Build history of the part. All positions in model axes, mm. A direction names the side the tool comes from. Coordinates: 2 decimals unless noted, no trailing zeros. Loops run counter-clockwise (first coordinate to the right, second up) from the corner with the lowest first, then second, coordinate; pieces in that order, holes last. Notation, with made-up numbers: (19.5, -33) -> (45.5, -33) arc R15 cw to (45.5, -29) -> close; hole circle Ø10 at (2, 41). An arc over 180 degrees is marked (long way). One line per item, written item: value. Start each with the question number.
Autodesk Inventor part; units mm, degrees
ref_plane "YZ Plane" through (0, 0, 0) normal (1, 0, 0) x (0, 1, 0)
ref_plane "XZ Plane" through (0, 0, 0) normal (0, 1, 0) x (-1, 0, 0)
ref_plane "XY Plane" through (0, 0, 0) normal (0, 0, 1) x (1, 0, 0)
sketch "Boceto1" plane through (0, 0, 0) normal (0, 1, 0) x (-1, 0, 0)
  line L0 (0, 0) -> (0, -22)
  line L1 (0, -22) -> (0, -23)
  line L2 (0, 0) -> (15, 0)
  line L3 (0, -23) -> (15, -23)
  line L4 (15, -23) -> (15, -27)
  line L5 (15, -27) -> (-4, -27)
  line L6 (-4, -27) -> (-4, 0)
  line L7 (-4, 0) -> (-4, 4)
  line L8 (-4, 4) -> (15, 4)
  line L9 (15, 4) -> (15, 0)
  line L10 (15, 4) -> (10, 4)
  line L11 (10, 4) -> (-4, 2)
  line L12 (15, -27) -> (10, -27)
  line L13 (10, -27) -> (-4, -25.6809)
  dimension "d0" = 22
  dimension "d1" = 1
  dimension "d2" = 15
  dimension "d3" = 15
  dimension "d4" = 4
  dimension "d5" = 19
  dimension "d6" = 4
  dimension "d7" = 5
  dimension "d8" = 5
extrude "Extrusión1" add sketch "Boceto1" along normal blind 12 contours L0 L1 L3 L4 L5 L13 L6 L7 L11 L8 L9 L2
sketch "Boceto2" plane through (-15, 0, 0) normal (-1, 0, 0) x (0, 0, 1)
  line L0 (4, 0) -> (4, 12)
  line L1 (4, 6) -> (-27, 6)
  line L2 (-27, 0) -> (-27, 12)
  line L3 (4, 6) -> (3, 6)
  circle A0 centre (3, 6) radius 1
  line L4 (-27, 6) -> (-26, 6)
  circle A1 centre (-26, 6) radius 1
  point P0 (0, 0)
  dimension "d11" = 1
  dimension "d12" = 1
extrude "Extrusión2" cut sketch "Boceto2" against normal blind 12
sketch "Boceto3" plane through (0, 12, 0) normal (0, 1, 0) x (1, 0, 0)
  line L0 (-10, -4) -> (4, -2)
  line L1 (0, -2.5714) -> (-15, -2.5714)
  line L2 (-15, -2) -> (-3, -2)
  line L3 (-15, -2.5714) -> (-13, -2.5714)
  line L4 (-13, -2.5714) -> (-13, -4)
  line L5 (-15, -4) -> (-10, -4)
  line L6 (-13, -4) -> (-10.0485, -4)
  line L7 (-10.0485, -4) -> (0, -2.5714)
  line L8 (-10, 27) -> (-15, 27)
  line L9 (-15, 27) -> (-13, 27)
  line L10 (-13, 27) -> (-13, 25.6179)
  line L11 (-13, 25.6179) -> (-3.0681, 25.6179)
  line L12 (-10, 27) -> (-3, 26.3405)
  line L13 (-3.0681, 25.6179) -> (-3, 26.3405)
  line L14 (-3, 26.3405) -> (-13, 27)
  line L15 (-13, 27) -> (-10, 27)
  line L16 (-10, 27) -> (-3, 26.3405)
  line L17 (4, 25.6809) -> (-10, 27)
  point P0 (0, 0)
  dimension "d15" = 2
  dimension "d16" = 2
extrude "Extrusión3" cut sketch "Boceto3" against normal blind 12 contours L7 L5 L4 L1 | L12 L14 L8 | L14 L13 L11 L10
sketch "Boceto4" plane through (0, 12, 0) normal (0, 1, 0) x (1, 0, 0)
  line L0 (-10, -4) -> (0, -2.5714)
  line L1 (0, -2.5714) -> (-11.0485, -2.5714)
  line L2 (-15, -2) -> (-3, -2)
  line L3 (-11.0485, -2.5714) -> (-10.6007, -6.2769)
  line L4 (0, -2.5714) -> (4, -2)
  line L5 (-10.6007, -6.2769) -> (0, -2.5714)
  point P0 (0, 0)
extrude "Extrusión4" cut sketch "Boceto4" against normal blind 12
properties part number "test pinza"
Item 1: Tool access for faces 4 (the face through (-7, 6, -23)), 5 (the face through (-13, 2, 3)), 6 (the face through (-13, 9, -26)): list every direction of +Z, -Z, +X, -X, +Y, -Y with a clear straight run to the whole face (end or side of a thin tool).
Item 2: Drop flat-ended pins along their axis: pin 1 Ø0.5 at (y, z) = (6, 2.5) entering from -X; pin 2 Ø3.5 at (x, y) = (-3.5, 3.5) entering from +Z; pin 3 Ø1.6 at (y, z) = (10, 3.5) entering from +X. Give the stop position or say it passes through.
Item 3: Band-saw the part on C-C, the plane y = 6.5. List the corners of the cut face in (x, z), and give its area (3 significant figures).
Item 4: Band-saw the part on D-D, the plane y = 1.75. List the corners of the cut face in (x, z), and give its area (3 significant figures).
Item 5: Probe probe 1 along Z at (x, y) = (-10.5, 3); probe 2 along Z at (x, y) = (-11.75, 6); probe 3 along X at (y, z) = (10.5, -5). List the from-to ranges inside material, lowest first.
Item 6: Two-plate mould, pull along Z, no slides. Class faces 1 (the face through (-7, 6, 0)), 2 (the face through (-3, 6, -26)), 3 (the face through (-14, 9, 4)): +Z half, -Z half, draft (parallel to the pull), parting line (faces both ways), or undercut.
Item 7: Band-saw the part on A-A, the plane z = 3. List the corners of the cut face in (x, y), and give its area (3 significant figures).
Item 8: Band-saw the part on B-B, the plane x = -5.5. List the corners of the cut face in (y, z).
Worked out:
1. face 4: -X, +Y, -Y
1. face 5: +Z, +X, +Y, -Y
1. face 6: -Z, +Y, -Y
2. pin 1: stops at x = -3
2. pin 2: stops at z = 2.57
2. pin 3: stops at x = -13
3. outline: (-15, -27) -> (-13, -27) -> (-13, -26.87) -> (-15, -26.87) -> close; (-15, -25.13) -> (-3, -25.13) -> (-3, -26.34) -> (4, -25.68) -> (4, 2) -> (0, 2.57) -> (-3, 2.57) -> (-3, 2.13) -> (-15, 2.13) -> (-15, 0) -> (0, 0) -> (0, -23) -> (-15, -23) -> close; (-15, 3.87) -> (-13, 3.87) -> (-13, 4) -> (-15, 4) -> close
3. area: 182 mm²
4. outline: (-15, -27) -> (-13, -27) -> (-13, -25.62) -> (-3.07, -25.62) -> (-3, -26.34) -> (4, -25.68) -> (4, 2) -> (0, 2.57) -> (-13, 2.57) -> (-13, 4) -> (-15, 4) -> (-15, 0) -> (0, 0) -> (0, -23) -> (-15, -23) -> close
4. area: 198 mm²
5. probe 1: z = -25.62 to -23, 0 to 2.57
5. probe 2: z = -25 to -23, 0 to 2
5. probe 3: x = 0 to 4
6. face 1: undercut
6. face 2: draft
6. face 3: +Z half
7. outline: (-15, 0) -> (-13, 0) -> (-13, 5) -> (-15, 5) -> close; (-15, 7) -> (-13, 7) -> (-13, 12) -> (-15, 12) -> close
7. area: 20.0 mm²
8. outline: (0, -25.62) -> (5.08, -25.62) arc R1 cw to (6.92, -25.62) -> (12, -25.62) -> (12, -23) -> (0, -23) -> close; (0, 0) -> (12, 0) -> (12, 2.57) -> (6.9, 2.57) arc R1 cw to (5.1, 2.57) -> (0, 2.57) -> close
